from build123d import *

# Parameters (mm, degrees)
CUT_EXTRUDE1_REACH  = 134.808
SKETCH3_R           = 5.1
BOSS_EXTRUDE3_DEPTH = 20
CUT_EXTRUDE2_REACH  = 202.893
SKETCH6_R           = 3.25
CIRPATTERN1_COUNT   = 6


with BuildPart() as part:
    # Sketch1 → Revolve1 (revolve)
    with BuildSketch(Plane(origin=(0, 0, 0), x_dir=(1, 0, 0), z_dir=(0, 1, 0))):
        with BuildLine():
            Line((0, 0), (82, 0))
            Line((82, 0), (82, -30))
            Line((82, -30), (87, -30))
            Line((87, -30), (87, -50))
            Line((87, -50), (70, -50))
            Line((70, -50), (70, -15))
            ThreePointArc((70, -15), (68.535533906, -11.464466094), (65, -10))
            Line((65, -10), (0, -10))
            Line((0, -10), (0, 0))
        make_face()
    revolve(axis=Axis((0, 0, 0), (0, 0, -1)))

    # Sketch3 → Cut-Extrude1 (cut, up to next)
    with BuildSketch(Plane(origin=(0, 0, 0), x_dir=(-1, 0, 0), z_dir=(0, 0, -1)), mode=Mode.PRIVATE) as cut_extrude1_sk1:
        with Locations((-25, 0)):
            Circle(SKETCH3_R)
    cut_extrude1_tool1 = extrude(cut_extrude1_sk1.sketch, amount=-CUT_EXTRUDE1_REACH, mode=Mode.PRIVATE) & part.part
    # Sketch3 → Cut-Extrude1 (cut, up to next)
    with BuildSketch(Plane(origin=(0, 0, 0), x_dir=(-1, 0, 0), z_dir=(0, 0, -1)), mode=Mode.PRIVATE) as cut_extrude1_sk2:
        with Locations((25, 0)):
            Circle(SKETCH3_R)
    cut_extrude1_tool2 = extrude(cut_extrude1_sk2.sketch, amount=-CUT_EXTRUDE1_REACH, mode=Mode.PRIVATE) & part.part
    # Sketch3 → Cut-Extrude1 (cut, up to next)
    with BuildSketch(Plane(origin=(0, 0, 0), x_dir=(-1, 0, 0), z_dir=(0, 0, -1)), mode=Mode.PRIVATE) as cut_extrude1_sk3:
        with BuildLine():
            ThreePointArc((10.592538838, 60.073272934), (15.22636256, 63.317911235), (11.981724259, 67.951734958))
            ThreePointArc((11.981724259, 67.951734958), (0, 69), (-11.981724259, 67.951734958))
            ThreePointArc((-11.981724259, 67.951734958), (-15.22636256, 63.317911235), (-10.592538838, 60.073272934))
            ThreePointArc((-10.592538838, 60.073272934), (0, 61), (10.592538838, 60.073272934))
        make_face()
    cut_extrude1_tool3 = extrude(cut_extrude1_sk3.sketch, amount=-CUT_EXTRUDE1_REACH, mode=Mode.PRIVATE) & part.part
    add(cut_extrude1_tool1.solids().sort_by_distance((25, 0, 0))[0], mode=Mode.SUBTRACT)
    add(cut_extrude1_tool2.solids().sort_by_distance((-25, 0, 0))[0], mode=Mode.SUBTRACT)
    add(cut_extrude1_tool3.solids().sort_by_distance((0, 64.527802, 0))[0], mode=Mode.SUBTRACT)

    # Sketch5 → Boss-Extrude3 (add)
    with BuildSketch(Plane.XY.offset(50)):
        Polygon((80, 10), (80, 0), (80, -10), (70, -10), (70, 10), align=None)
    boss_extrude3 = extrude(amount=BOSS_EXTRUDE3_DEPTH)

    # Sketch6 → Cut-Extrude2 (cut, up to next)
    with BuildSketch(Plane(origin=(80, 0, 0), x_dir=(0, 1, 0), z_dir=(-1, 0, 0)), mode=Mode.PRIVATE) as cut_extrude2_sk1:
        with Locations(Location((0, -60, 0), (0, 0, 90))):
            Circle(SKETCH6_R)
    cut_extrude2_tool1 = extrude(cut_extrude2_sk1.sketch, amount=CUT_EXTRUDE2_REACH, mode=Mode.PRIVATE) & part.part
    cut_extrude2 = cut_extrude2_tool1.solids().sort_by_distance((80, 0, 60))[0]
    add(cut_extrude2, mode=Mode.SUBTRACT)

    # CirPattern1: Boss-Extrude3, Cut-Extrude2 ×6 about axis
    cirpattern1_axis = Axis((0, 0, 0), (0, 0, 1))
    add([boss_extrude3.rotate(cirpattern1_axis, i * 360 / CIRPATTERN1_COUNT) for i in range(1, CIRPATTERN1_COUNT)])
    add([cut_extrude2.rotate(cirpattern1_axis, i * 360 / CIRPATTERN1_COUNT) for i in range(1, CIRPATTERN1_COUNT)], mode=Mode.SUBTRACT)


solid = part.part
Could you check a few things on this model? Use its own coordinates, in mm. A direction names the side the tool comes from. Give positions to 0.01 mm unless a question says otherwise; leave off trailing zeros. Order: outer loops, then holes, each group sorted by start corner. A loop starts at its lowest first (then second) coordinate and runs counter-clockwise, first axis right, second up. Notation, with made-up numbers: (24, 17.5) - (72, 17.5) arc R25 ccw to (72, 33.5) - close; hole circle Ø8 at (39.25, 41.5). An arc over 180 degrees is marked (long way). One line per question, with ' | ' between items. Start each with the question number.
Item 1: I need wall thicknesses on probe 1 along X at (y, z) = (0, 26); probe 2 along X at (y, z) = (-64.5, 61). Which ranges of each line are inside material? Lowest first, please. Write a range as [from, to].
Item 2: Thinking about a two-plate mould opening in X: for faces 1 (the flat face through (75, -10, 60)), 2 (the flat face through (-39.88, 69.35, 55.42)), 3 (the cylindrical face through (-15.21, 63.23, 5.92)), which applies, pulls with the +X half, pulls with the -X half, needs draft (parallel to the pull), parting line crosses it, or undercut?
Item 3: I want a section at B-B on z = 24. Write out the boundary of the cut face in (x, y).
Item 4: For faces 4 (the flat face through (-80, 0, 55)), 5 (the flat face through (46.195, 60.013, 59.86)), 6 (the flat face through (-46.125, 59.891, 59.86)), 7 (the flat face through (34.88, -60.69, 55.42)), which set-ups out of +Z, -Z, +X, -X, +Y, -Y let a thin tool reach every point of the face, with its end or its side?
Item 5: I want a section at C-C on z = 60. Give the number of separate pieces and of enclosed holes in the cut face, then the cut area to 3 significant figures.
Item 6: I'm going to push flat-ended pins straight in: pin 1 Ø5 at (x, z) = (-46.5, 47.5) entering from -Y; pin 2 Ø22 at (y, z) = (3, 57.5) entering from +X; pin 3 Ø8 at (x, z) = (74, 62) entering from -Y; pin 4 Ø4 at (y, z) = (37.5, 46) entering from -X. Where does each tip first touch, or does it pass through?
Item 7: I want a section at A-A on x = 0. Write out the boundary of the cut face in (y, z), then the cut area to 3 significant figures.
Verdict:
1) probe 1: [-82, -70], [70, 82] | probe 2: [-48.28, -40.81], [-33.67, -28.28], [28.28, 33.67], [40.81, 48.28]
2) face 1: needs draft | face 2: pulls with the -X half | face 3: undercut
3) outline: circle Ø164 at (0, 0); hole circle Ø140 at (0, 0)
4) face 4: +Z, -X, +Y, -Y | face 5: +Z, +X | face 6: +Z, -X | face 7: +Z
5) separate pieces: 12 | enclosed holes: 0 | area: 810 mm^2
6) pin 1: y = -75.05 | pin 2: x = 87 | pin 3: y = -10 | pin 4: x = -79.43
7) outline: (-87, 30) - (-82, 30) - (-82, 0) - (61, 0) - (61, 10) - (-65, 10) arc R5 cw to (-70, 15) - (-70, 50) - (-87, 50) - close; (69, 0) - (82, 0) - (82, 30) - (87, 30) - (87, 50) - (70, 50) - (70, 15) arc R5 cw to (69, 12) - close | area: 2,730 mm^2
